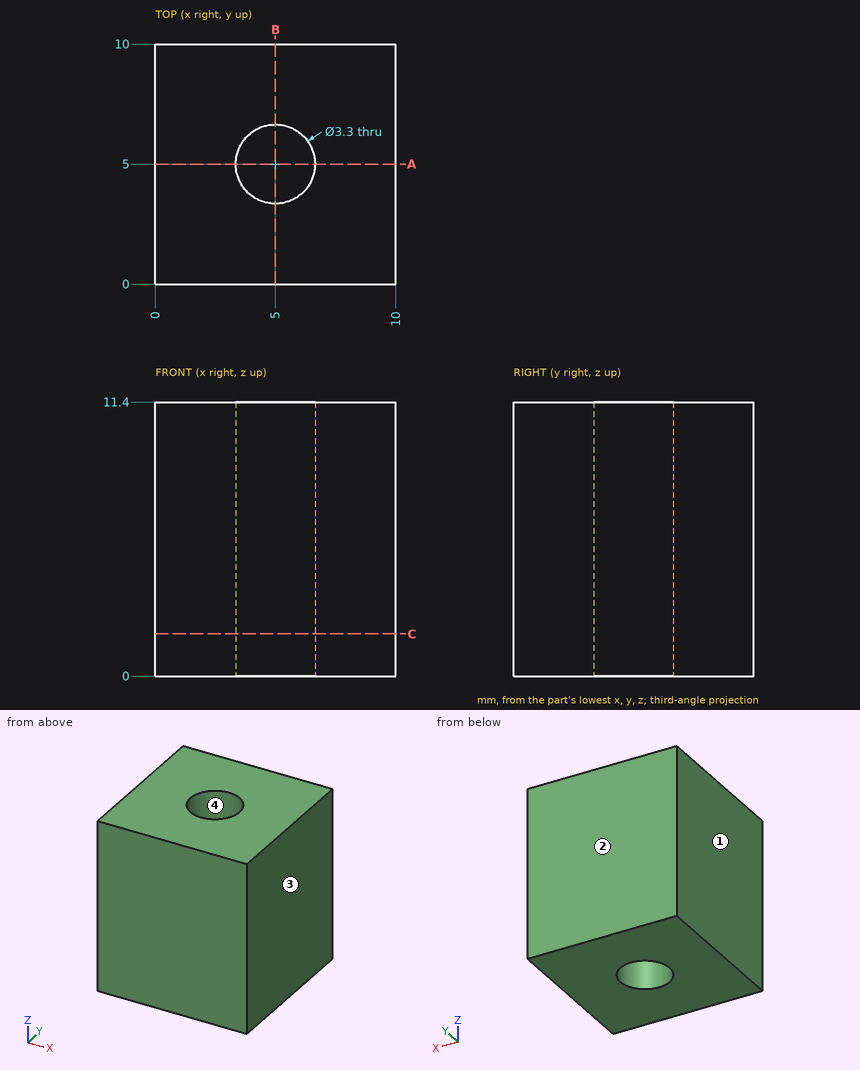
The figure shows three views and two pictorial views of one solid part (mm, origin at its lowest corner). Answer the questions. Give positions to 0.01 mm unless a question says otherwise; leave off trailing zeros. Write each loop counter-clockwise with the first axis right and the second up, starting at its lowest first coordinate (ties: lowest second). Pieces come first, ordered by that corner, then holes. Notation, with made-up numbers: (41.5, 74.5) - (78.5, 74.5) arc R15 ccw to (78.5, 83.5) - close; hole circle Ø11 at (34, 10). An arc over 180 degrees is marked (long way). Use one line per item in the form item = value. Start each with the question number.
1) Consider line 1 along Y through (x, z) = (5, 7.5); line 2 along X through (y, z) = (4.75, 3); line 3 along X through (y, z) = (6.5, 2.5). Determine where each line is inside the solid, lowest interval first. Write a range as from..to.
2) Flat-ended cylindrical pins translate along their axes: pin 1 Ø2 at (x, y) = (5, 5) entering from -Z; pin 2 Ø6 at (x, y) = (2.5, 7.5) entering from -Z. Find the tip coordinate at first contact, or state that the pin passes through.
3) Find section C-C on z = 1.75. Determine the outline of the cut face in (x, y).
4) The mould has two halves that part along X. Classify the marked faces 1, 2, 3 and 4: pulls with the +X half, pulls with the -X half, needs draft (parallel to the pull), parting line crosses it, or undercut.
5) Find section A-A on y = 5. Determine the outline of the cut face in (x, z).
Geometry results:
q1.line_1 = 0..3.35, 6.65..10
q1.line_2 = 0..3.37, 6.63..10
q1.line_3 = 0..4.31, 5.69..10
q2.pin_1 = through
q2.pin_2 = 0
q3.outline = (0, 0) - (10, 0) - (10, 10) - (0, 10) - close; hole circle Ø3.3 at (5, 5)
q4.face_1 = pulls with the -X half
q4.face_2 = needs draft
q4.face_3 = pulls with the +X half
q4.face_4 = undercut
q5.outline = (0, 0) - (3.35, 0) - (3.35, 11.4) - (0, 11.4) - close; (6.65, 0) - (10, 0) - (10, 11.4) - (6.65, 11.4) - close
